Can you work these out from the model? Positions are in its coordinate system, mm. Give positions to 0.01 mm unless a question says otherwise; leave off trailing zeros. Order: outer loops, then holes, each group sorted by start corner. A loop starts at its lowest first (then second) coordinate and runs counter-clockwise, first axis right, second up. Notation, with made-up numbers: (86.25, 71.25) - (144.25, 71.25) arc R22 ccw to (144.25, 107.25) - close; hole circle Ø7 at (-34.75, -30). An arc over 180 degrees is marked (long way). Return JSON: item names as keys, results as strings.
```python
from build123d import *

# Parameters (mm, degrees)
SKETCH1_R           = 3
BOSS_EXTRUDE1_DEPTH = 2
BOSS_EXTRUDE4_DEPTH = 2
SKETCH4_R           = 0.5
CUT_EXTRUDE1_DEPTH  = 2


with BuildPart() as part:
    # Sketch1 → Boss-Extrude1 (new body)
    with BuildSketch(Plane(origin=(0, 0, 0), x_dir=(1, 0, 0), z_dir=(0, 1, 0))):
        Circle(SKETCH1_R)
    extrude(amount=BOSS_EXTRUDE1_DEPTH)

    # Sketch3 → Boss-Extrude4 (add)
    with BuildSketch(Plane(origin=(0, 2, 0), x_dir=(1, 0, 0), z_dir=(0, 1, 0))):
        with BuildLine():
            ThreePointArc((-2.992341362, 0.214226915), (9.2675e-05, -2.999999999), (2.992328121, 0.214411791))
            Line((2.992328121, 0.214411791), (1.998320796, 27.995599459))
            ThreePointArc((1.998320796, 27.995599459), (-0.000428771, 29.924085477), (-1.999123301, 27.995542419))
            Line((-1.999123301, 27.995542419), (-2.992341362, 0.214226915))
        make_face()
    extrude(amount=-BOSS_EXTRUDE4_DEPTH)

    # Sketch4 → Cut-Extrude1 (cut)
    with BuildSketch(Plane(origin=(0, 2, 0), x_dir=(1, 0, 0), z_dir=(0, 1, 0))):
        with Locations((-0.000203324, 14.190099999)):
            Circle(SKETCH4_R)
        with Locations((-6.6844e-05, 4.6651)):
            Circle(SKETCH4_R)
    extrude(amount=-CUT_EXTRUDE1_DEPTH, mode=Mode.SUBTRACT)


solid = part.part
```
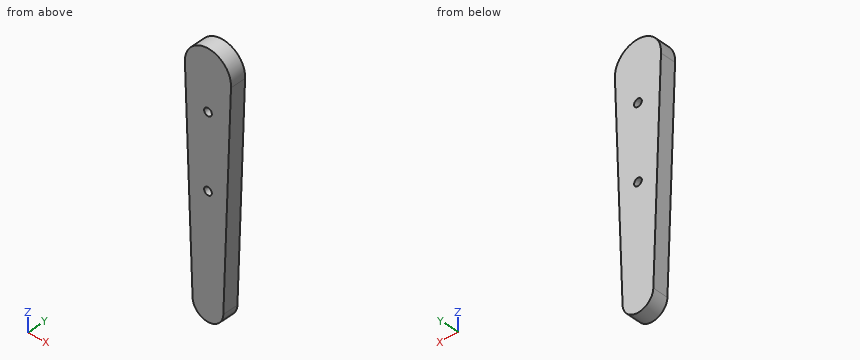
1. If I drill on L1, parallel to Z at x = 0.4, y = 1.5; L2, parallel to Z at x = -0.2, y = 1.8; L3, parallel to X at y = 1.2, z = -28, over which ranges is the centre line in solid material (lowest first)? Write a range as [from, to].
Checks:
{"L1": "[-29.88, -14.49], [-13.89, -4.97], [-4.37, 2.97]", "L2": "[-29.91, -14.65], [-13.73, -5.12], [-4.21, 2.99]", "L3": "[-2, 2]"}
2. Suppose I cut it at D-D (x = -1.4). List the corners of the cut face in (y, z) for me.
Checks:
{"outline": "(0, -29.35) - (2, -29.35) - (2, 2.65) - (0, 2.65) - close"}
3. Suppose I cut it at B-B (y = 1.55). List the corners of the cut face in (x, z) for me, plus the area to 3 significant figures.
Checks:
{"outline": "(-2.99, -0.21) - (-2, -28) arc R2 ccw to (2, -28) - (2.99, -0.21) arc R3 ccw (long way) to start; hole circle Ø1 at (0, -14.19); hole circle Ø1 at (0, -4.67)", "area": "159 mm^2"}
4. Suppose I cut it at A-A (x = 0). List the corners of the cut face in (y, z) for me, plus the area to 3 significant figures.
Checks:
{"outline": "(0, -29.92) - (2, -29.92) - (2, -14.69) - (0, -14.69) - close; (0, -13.69) - (2, -13.69) - (2, -5.17) - (0, -5.17) - close; (0, -4.17) - (2, -4.17) - (2, 3) - (0, 3) - close", "area": "61.8 mm^2"}
5. Suppose I cut it at C-C (z = -13). List the corners of the cut face in (x, y) for me, plus the area to 3 significant figures.
Checks:
{"outline": "(-2.54, 0) - (2.53, 0) - (2.53, 2) - (-2.54, 2) - close", "area": "10.1 mm^2"}
